Autodesk Inventor part; units mm, degrees
ref_plane "YZ Plane" through (0, 0, 0) normal (1, 0, 0) x (0, 1, 0)
ref_plane "XZ Plane" through (0, 0, 0) normal (0, 1, 0) x (-1, 0, 0)
ref_plane "XY Plane" through (0, 0, 0) normal (0, 0, 1) x (1, 0, 0)
sketch "Sketch3" plane through (0, 0, 0) normal (0, 0, 1) x (1, 0, 0)
  line L0 (0, 0) -> (-80, 0)
  line L1 (-80, 0) -> (-80, 80)
  line L2 (-80, 80) -> (0, 80)
  line L3 (0, 80) -> (0, 0)
  line L4 (-75, 75) -> (-5, 75)
  line L5 (-5, 75) -> (-5, 5)
  line L6 (-5, 5) -> (-75, 5)
  line L7 (-75, 5) -> (-75, 75)
  dimension "d129" = 80
  dimension "d130" = 80
  dimension "d131" = 70
  dimension "d132" = 70
extrude "Extrusion19" add sketch "Sketch3" along normal blind 68
sketch "Sketch18" plane through (0, 0, 68) normal (0, 0, 1) x (1, 0, 0)
  line L0 (0, 80) -> (-80, 80)
  line L1 (0, 0) -> (-80, 0)
  line L2 (-80, 0) -> (-80, 80)
  line L3 (-80, 80) -> (0, 80)
  line L4 (0, 80) -> (0, 0)
  dimension "d135" = 80
  dimension "d136" = 80
extrude "Extrusion20" add sketch "Sketch18" along normal blind 4
sketch "Sketch20" plane through (0, 0, 72) normal (0, 0, 1) x (1, 0, 0)
  line L0 (-67.5, 67.5) -> (-12.5, 67.5)
  line L1 (-12.5, 67.5) -> (-12.5, 12.5)
  line L2 (-12.5, 12.5) -> (-67.5, 12.5)
  line L3 (-67.5, 12.5) -> (-67.5, 67.5)
  point P0 (0, 0)
  dimension "d139" = 55
  dimension "d140" = 55
extrude "Extrusion21" cut sketch "Sketch20" against normal blind 2
sketch "Sketch21" plane through (0, 0, 0) normal (1, 0, 0) x (0, 0, -1)
  line L0 (-63.5, 12.5) -> (-8.5, 12.5)
  line L1 (-8.5, 12.5) -> (-8.5, 67.5)
  line L2 (-8.5, 67.5) -> (-63.5, 67.5)
  line L3 (-63.5, 67.5) -> (-63.5, 12.5)
  point P0 (0, 0)
  dimension "d143" = 55
  dimension "d144" = 55
sketch "Sketch22" plane through (-80, 0, 0) normal (-1, 0, 0) x (0, 0, 1)
  line L0 (8.5, 12.5) -> (63.5, 12.5)
  line L1 (63.5, 12.5) -> (63.5, 67.5)
  line L2 (63.5, 67.5) -> (8.5, 67.5)
  line L3 (8.5, 67.5) -> (8.5, 12.5)
  point P0 (0, 0)
  dimension "d145" = 55
  dimension "d146" = 55
sketch "Sketch23" plane through (-80, 0, 0) normal (0, -1, 0) x (1, 0, 0)
  line L0 (12.5, 8.5) -> (67.5, 8.5)
  line L1 (67.5, 8.5) -> (67.5, 63.5)
  line L2 (67.5, 63.5) -> (12.5, 63.5)
  line L3 (12.5, 63.5) -> (12.5, 8.5)
  point P0 (80, 0)
  dimension "d147" = 55
  dimension "d148" = 55
sketch "Sketch24" plane through (-80, 80, 0) normal (0, 1, 0) x (1, 0, 0)
  line L0 (12.5, -8.5) -> (67.5, -8.5)
  line L1 (67.5, -8.5) -> (67.5, -63.5)
  line L2 (67.5, -63.5) -> (12.5, -63.5)
  line L3 (12.5, -63.5) -> (12.5, -8.5)
  point P0 (80, 0)
  dimension "d149" = 55
  dimension "d150" = 55
extrude "Extrusion22" cut sketch "Sketch21" against normal blind 2
extrude "Extrusion23" cut sketch "Sketch24" against normal blind 2
extrude "Extrusion24" cut sketch "Sketch23" against normal blind 2
extrude "Extrusion25" cut sketch "Sketch22" against normal blind 2
sketch "Sketch25" plane through (-80, 0, 0) normal (0, -1, 0) x (1, 0, 0)
  line L0 (80, 0) -> (0, 0)
  line L1 (0, 0) -> (10.6, 0)
  line L2 (10.6, 0) -> (10.6, 5.6)
  line L3 (10.6, 5.6) -> (0, 5.6)
  line L4 (0, 5.6) -> (0, 0)
  line L5 (80, 0) -> (69.4, 0)
  line L6 (69.4, 0) -> (69.4, 5.6)
  line L7 (69.4, 5.6) -> (80, 5.6)
  line L8 (80, 5.6) -> (80, 0)
  dimension "d159" = 10.6
  dimension "d160" = 5.6
  dimension "d161" = 10.6
  dimension "d162" = 5.6
properties part number "End-Effector"
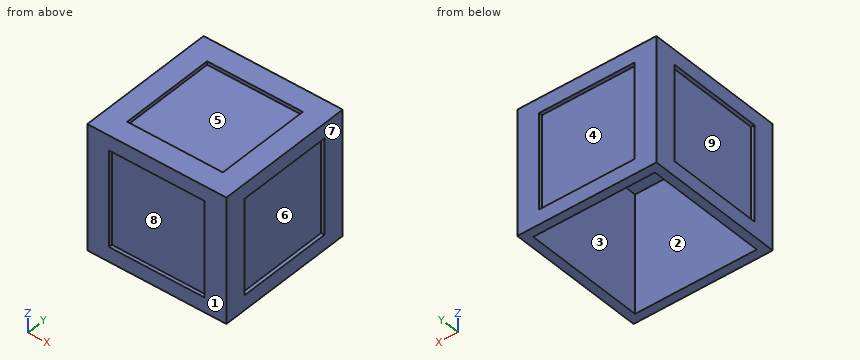
Source: CAD feature listing. Evaluate the final solid. Frame: model axes, mm. Face numbers are marked on the shaded views. A direction names the side the tool comes from. Give positions to 0.01 mm unless a question says otherwise; leave off trailing zeros. Write each loop counter-clockwise with the first axis right and the second up, starting at its lowest first coordinate (ties: lowest second). Pieces come first, ordered by that corner, then holes. Notation, with made-up numbers: (64.25, 48) - (100.25, 48) arc R27 cw to (100.25, 68) - close; hole circle Ø8 at (24, -9). An arc over 180 degrees is marked (long way). Write item = value, one per line. Start each with the question number.
Q1. Pin query (flat end, axial travel): pin 1 Ø2 at (x, z) = (-23.5, 50.5) entering from -Y; pin 2 Ø6 at (y, z) = (32.5, 25) entering from +X; pin 3 Ø10 at (x, y) = (-17, 17.5) entering from -Z. Return the tip coordinate at first contact, or that it passes through.
Q2. Material intervals for probe 1 along X at (y, z) = (72.5, 3); probe 2 along Y at (x, z) = (-56, 55); probe 3 along Y at (x, z) = (-73.5, 31), sorted ascending.
Q3. Cut plane B-B, the plane z = 20.5. Return loops of the section in (x, y).
Q4. Draft query along Y for the marked faces 1, 2, 3 and 4. Return one class per face: +Y half, -Y half, draft (parallel to the pull), parting line (faces both ways), or undercut.
Q5. Reachability of the marked faces 5, 6, 7, 8 and 9 from +Z, -Z, +X, -X, +Y, -Y: full face, straight path, thin tool, end or side. Return the list, or none.
Q6. Cut plane A-A, the plane y = 60. Return loops of the section in (x, z), then the cut area to 3 significant figures.
Q7. Cut plane C-C, the plane x = -65.5. Return loops of the section in (y, z).
Q8. Cut plane D-D, the plane y = 73. Return loops of the section in (x, z).
Computed values:
q1.pin_1 = 2
q1.pin_2 = -2
q1.pin_3 = 68
q2.probe_1 = -80 to -75, -5 to 0
q2.probe_2 = 2 to 5, 75 to 78
q2.probe_3 = 0 to 5, 75 to 80
q3.outline = (-80, 0) - (-67.5, 0) - (-67.5, 2) - (-12.5, 2) - (-12.5, 0) - (0, 0) - (0, 12.5) - (-2, 12.5) - (-2, 67.5) - (0, 67.5) - (0, 80) - (-12.5, 80) - (-12.5, 78) - (-67.5, 78) - (-67.5, 80) - (-80, 80) - (-80, 67.5) - (-78, 67.5) - (-78, 12.5) - (-80, 12.5) - close; hole (-75, 5) - (-5, 5) - (-5, 75) - (-75, 75) - close
q4.face_1 = -Y half
q4.face_2 = undercut
q4.face_3 = undercut
q4.face_4 = +Y half
q5.face_5 = +Z
q5.face_6 = +X
q5.face_7 = +Z, -Z, +X, +Y, -Y
q5.face_8 = -Y
q5.face_9 = -X
q6.outline = (-80, 0) - (-75, 0) - (-75, 68) - (-5, 68) - (-5, 0) - (0, 0) - (0, 8.5) - (-2, 8.5) - (-2, 63.5) - (0, 63.5) - (0, 72) - (-12.5, 72) - (-12.5, 70) - (-67.5, 70) - (-67.5, 72) - (-80, 72) - (-80, 63.5) - (-78, 63.5) - (-78, 8.5) - (-80, 8.5) - close
q6.area = 670 mm²
q7.outline = (0, 0) - (5, 0) - (5, 68) - (75, 68) - (75, 0) - (80, 0) - (80, 8.5) - (78, 8.5) - (78, 63.5) - (80, 63.5) - (80, 72) - (67.5, 72) - (67.5, 70) - (12.5, 70) - (12.5, 72) - (0, 72) - (0, 63.5) - (2, 63.5) - (2, 8.5) - (0, 8.5) - close
q8.outline = (-80, 0) - (-75, 0) - (-75, 68) - (-5, 68) - (-5, 0) - (0, 0) - (0, 72) - (-80, 72) - close
